Work out the finished part from the listing and answer in its coordinate system (mm). Give positions to 0.01 mm unless a question says otherwise; leave off trailing zeros. Loops run counter-clockwise (first coordinate to the right, second up) from the corner with the lowest first, then second, coordinate; pieces in that order, holes last. Notation, with made-up numbers: (0, 42) - (29, 42) arc R28 cw to (29, 63) - close; hole circle Ø5 at (-7, -35.75). An arc over 180 degrees is marked (long way). One line per question, with ' | ' between items.
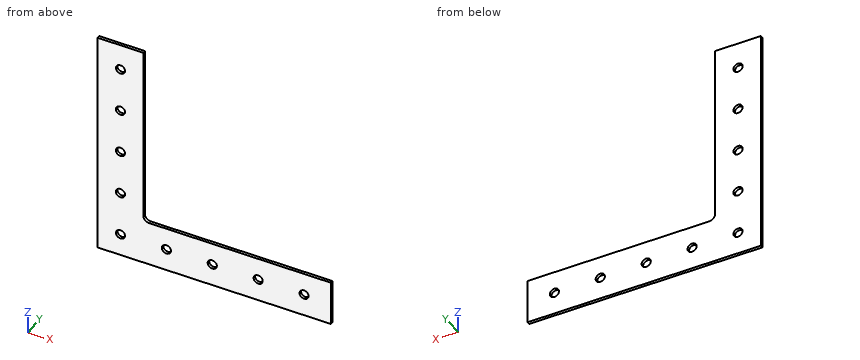
Autodesk Inventor part; units mm, degrees
ref_plane "YZ Plane" through (0, 0, 0) normal (1, 0, 0) x (0, 1, 0)
ref_plane "XZ Plane" through (0, 0, 0) normal (0, 1, 0) x (-1, 0, 0)
ref_plane "XY Plane" through (0, 0, 0) normal (0, 0, 1) x (1, 0, 0)
sketch "Sketch1" plane through (0, 0, 0) normal (0, 1, 0) x (-1, 0, 0)
  line L0 (0, 0) -> (-25.4, 0)
  line L1 (-25.4, -35.921) -> (-25.4, -127)
  line L2 (-25.4, -152.4) -> (0, -152.4)
  line L3 (0, -152.4) -> (0, 0)
  line L4 (0, -152.4) -> (-152.4, -152.4)
  line L5 (-152.4, -152.4) -> (-152.4, -127)
  line L6 (-116.479, -127) -> (-25.4, -127)
  line L7 (0, -127) -> (0, -152.4)
  line L8 (-152.4, -127) -> (-25.4, 0)
  line L9 (-25.4, -35.921) -> (-116.479, -127)
  dimension "d0" = 25.4
  dimension "d1" = 152.4
  dimension "d2" = 152.4
  dimension "d3" = 25.4
  dimension "d4" = 25.4
extrude "Extrusion1" add sketch "Sketch1" along normal blind 1.5875
sketch "Sketch2" plane through (0, 1.5875, 0) normal (0, 1, 0) x (1, 0, 0)
  line L0 (152.4, 152.4) -> (0, 152.4)
  line L1 (0, 152.4) -> (25.4, 152.4)
  line L2 (25.4, 35.921) -> (25.4, 127)
  line L3 (25.4, 152.4) -> (25.4, 127)
  line L4 (25.4, 127) -> (0, 152.4)
  line L5 (25.4, 152.4) -> (0, 127)
  line L6 (0, 152.4) -> (0, 0)
  line L7 (12.7, 139.7) -> (38.1, 139.7)
  line L8 (38.1, 139.7) -> (63.5, 139.7)
  line L9 (63.5, 139.7) -> (88.9, 139.7)
  line L10 (88.9, 139.7) -> (114.3, 139.7)
  line L11 (114.3, 139.7) -> (139.7, 139.7)
  line L12 (12.7, 139.7) -> (12.7, 114.3)
  line L13 (12.7, 114.3) -> (12.7, 88.9)
  line L14 (12.7, 88.9) -> (12.7, 63.5)
  line L15 (12.7, 63.5) -> (12.7, 38.1)
  line L16 (12.7, 38.1) -> (12.7, 12.7)
  circle A0 centre (12.7, 139.7) radius 2.54
  circle A1 centre (38.1, 139.7) radius 2.54
  circle A2 centre (63.5, 139.7) radius 2.54
  circle A3 centre (88.9, 139.7) radius 2.54
  circle A4 centre (114.3, 139.7) radius 2.54
  circle A5 centre (139.7, 139.7) radius 2.54
  circle A6 centre (12.7, 114.3) radius 2.54
  circle A7 centre (12.7, 88.9) radius 2.54
  circle A8 centre (12.7, 63.5) radius 2.54
  circle A9 centre (12.7, 38.1) radius 2.54
  circle A10 centre (12.7, 12.7) radius 2.54
  dimension "d7" = 25.4
  dimension "d8" = 25.4
  dimension "d9" = 25.4
  dimension "d10" = 25.4
  dimension "d11" = 25.4
  dimension "d12" = 25.4
  dimension "d13" = 25.4
  dimension "d14" = 25.4
  dimension "d15" = 25.4
  dimension "d16" = 25.4
  dimension "d17" = 5.08
  dimension "d18" = 5.08
  dimension "d19" = 5.08
  dimension "d20" = 5.08
  dimension "d21" = 5.08
  dimension "d22" = 5.08
  dimension "d23" = 5.08
  dimension "d24" = 5.08
hole "Hole1" at (12.7, 1.5875, -139.7) at (38.1, 1.5875, -139.7) at (63.5, 1.5875, -139.7) at (88.9, 1.5875, -139.7) at (114.3, 1.5875, -139.7) at (12.7, 1.5875, -114.3) at (12.7, 1.5875, -88.9) at (12.7, 1.5875, -63.5) at (12.7, 1.5875, -38.1) direction (0, -1, 0) diameter 5.08 end through all
sketch "Sketch3" plane through (0, 1.5875, 0) normal (0, 1, 0) x (1, 0, 0)
  line L0 (116.479, 127) -> (25.4, 127)
  line L1 (116.479, 127) -> (129.179, 127)
  line L2 (129.179, 127) -> (129.179, 152.4)
  line L3 (152.4, 152.4) -> (0, 152.4)
  line L4 (25.4, 35.921) -> (25.4, 127)
  line L5 (25.4, 35.921) -> (25.4, 23.221)
  line L6 (25.4, 23.221) -> (0, 23.221)
  line L7 (0, 23.221) -> (0, 0)
  line L8 (25.4, 0) -> (152.4, 127)
  line L9 (0, 0) -> (25.4, 0)
  line L10 (25.4, 0) -> (152.4, 127)
  line L11 (152.4, 127) -> (152.4, 152.4)
  line L12 (152.4, 127) -> (152.4, 152.4)
  line L13 (152.4, 152.4) -> (129.179, 152.4)
  line L14 (116.479, 127) -> (25.4, 35.921)
  dimension "d32" = 12.7
  dimension "d33" = 12.7
extrude "Extrusion2" cut sketch "Sketch3" against normal blind 1.5875 contours L1 L2 L3 L11 L8 L9 L7 L6 L5 L14
sketch "Sketch4" plane through (0, 1.5875, 0) normal (0, 1, 0) x (1, 0, 0)
  line L0 (129.179, 127) -> (25.4, 127)
  line L1 (129.179, 127) -> (25.4, 23.221)
  line L2 (25.4, 59.142) -> (93.258, 127)
  line L3 (25.4, 127) -> (25.4, 23.221)
  line L4 (25.4, 59.142) -> (25.4, 23.221)
  point P0 (0, 0)
  dimension "d36" = 25.4
extrude "Extrusion3" add sketch "Sketch4" against normal blind 1.5875 contours L1 L3 L2 L0
fillet "Fillet1" radius 3.175 3 edges at (25.4, 0.7937, -127) (93.258, 0.7937, -127) (25.4, 0.7937, -59.142)
sketch "Sketch5" plane through (0, 1.5875, 0) normal (0, 1, 0) x (1, 0, 0)
  line L0 (25.4, 123.825) -> (25.4, 66.8072)
  line L1 (25.4, 23.221) -> (25.4, 123.825)
  line L2 (85.5928, 127) -> (28.575, 127)
  line L3 (28.575, 127) -> (135.0414, 127)
  line L4 (135.0414, 127) -> (135.0414, 23.221)
  line L5 (135.0414, 23.221) -> (25.4, 23.221)
  line L6 (28.575, 127) -> (85.5928, 127)
  line L7 (28.575, 127) -> (25.4, 123.825)
  point P0 (0, 0)
extrude "Extrusion4" cut sketch "Sketch5" against normal blind 25.4
properties part number "Gusset 2B 2.0"
1. Consider L1, parallel to Z at x = 12.7, y = 1.25; L2, parallel to X at y = 0.5, z = -139.7; L3, parallel to X at y = 0.85, z = -63.5. Determine where each line is inside the solid, lowest interval first.
Evaluation:
L1: -152.4 to -142.24, -137.16 to -116.84, -111.76 to -91.44, -86.36 to -66.04, -60.96 to -40.64, -35.56 to -23.22 | L2: 0 to 10.16, 15.24 to 35.56, 40.64 to 60.96, 66.04 to 86.36, 91.44 to 111.76, 116.84 to 129.18 | L3: 0 to 10.16, 15.24 to 25.4
2. Flat-ended cylindrical pins translate along their axes: pin 1 (3 mm diameter, centred on x = 27, z = -83, fed in from +Y); pin 2 (0.5 mm diameter, centred on x = 97, y = 0.5, fed in from +Z). Find the tip coordinate at first contact, or state that the pin passes through.
Evaluation:
pin 1: through | pin 2: z = -127
3. Find section A-A on x = 38.1. Write down the section's boundary in (y, z), then the cut area to 3 significant figures.
Evaluation:
outline: (0, -152.4) - (1.59, -152.4) - (1.59, -142.24) - (0, -142.24) - close; (0, -137.16) - (1.59, -137.16) - (1.59, -127) - (0, -127) - close | area: 32.3 mm2
4. Find section B-B on y = 1.1. State how many separate pieces and enclosed holes the cut face has, then the cut area to 3 significant figures.
Evaluation:
separate pieces: 1 | enclosed holes: 9 | area: 5,740 mm2
5. Find section C-C on z = -139.7. Write down the section's boundary in (x, y), then the cut area to 3 significant figures.
Evaluation:
outline: (0, 0) - (10.16, 0) - (10.16, 1.59) - (0, 1.59) - close; (15.24, 0) - (35.56, 0) - (35.56, 1.59) - (15.24, 1.59) - close; (40.64, 0) - (60.96, 0) - (60.96, 1.59) - (40.64, 1.59) - close; (66.04, 0) - (86.36, 0) - (86.36, 1.59) - (66.04, 1.59) - close; (91.44, 0) - (111.76, 0) - (111.76, 1.59) - (91.44, 1.59) - close; (116.84, 0) - (129.18, 0) - (129.18, 1.59) - (116.84, 1.59) - close | area: 165 mm2
6. Find section D-D on z = -63.5. Write down the section's boundary in (x, y), then the cut area to 3 significant figures.
Evaluation:
outline: (0, 0) - (10.16, 0) - (10.16, 1.59) - (0, 1.59) - close; (15.24, 0) - (25.4, 0) - (25.4, 1.59) - (15.24, 1.59) - close | area: 32.3 mm2
